Geometry: see drawing. Coordinates: mm, zero at the bounding-box minimum. Give positions to 0.01 mm unless a question says otherwise; leave off trailing zeros. Order: outer loops, then holes, each group sorted by start corner. A loop starts at its lowest first (then second) coordinate and runs counter-clockwise, first axis right, second up. Notation, with made-up numbers: M 2.5,74.25 L 12.5,74.25 A35 ccw 12.5,106.25 Z; hole C 39.25,12.25 d11. An arc over 180 degrees is marked long. Answer as a JSON object with one key per item and string values. Group by question number.
1. Section query C-C (x = 41.5). Output: boundary loops of the cut face in (y, z).
2. Material intervals for L1, parallel to X at y = 2.1, z = 21.5; L2, parallel to Z at x = 53.79, y = 0.9 (3 decimals); L3, parallel to Z at x = 26.5, y = 0.9, sorted ascending. Write a range as [from, to].
3. Section query A-A (x = 53.79). Output: boundary loops of the cut face in (y, z) (3 decimals).
4. Section query D-D (y = 1.7). Output: boundary loops of the cut face in (x, z) (3 decimals), plus the area to 3 significant figures.
5. Section query B-B (z = 6). Output: boundary loops of the cut face in (x, y).
6. Pin query (flat end, axial travel): P1, Ø1.6, axis at x = 22.5, y = 1, coming from the +Z side; P2, Ø1, axis at x = 32, y = 2, coming from the -Z side; P3, Ø1, axis at y = 1, z = 12, coming from the +X side. Return the tip coordinate at first contact, or that it passes through.
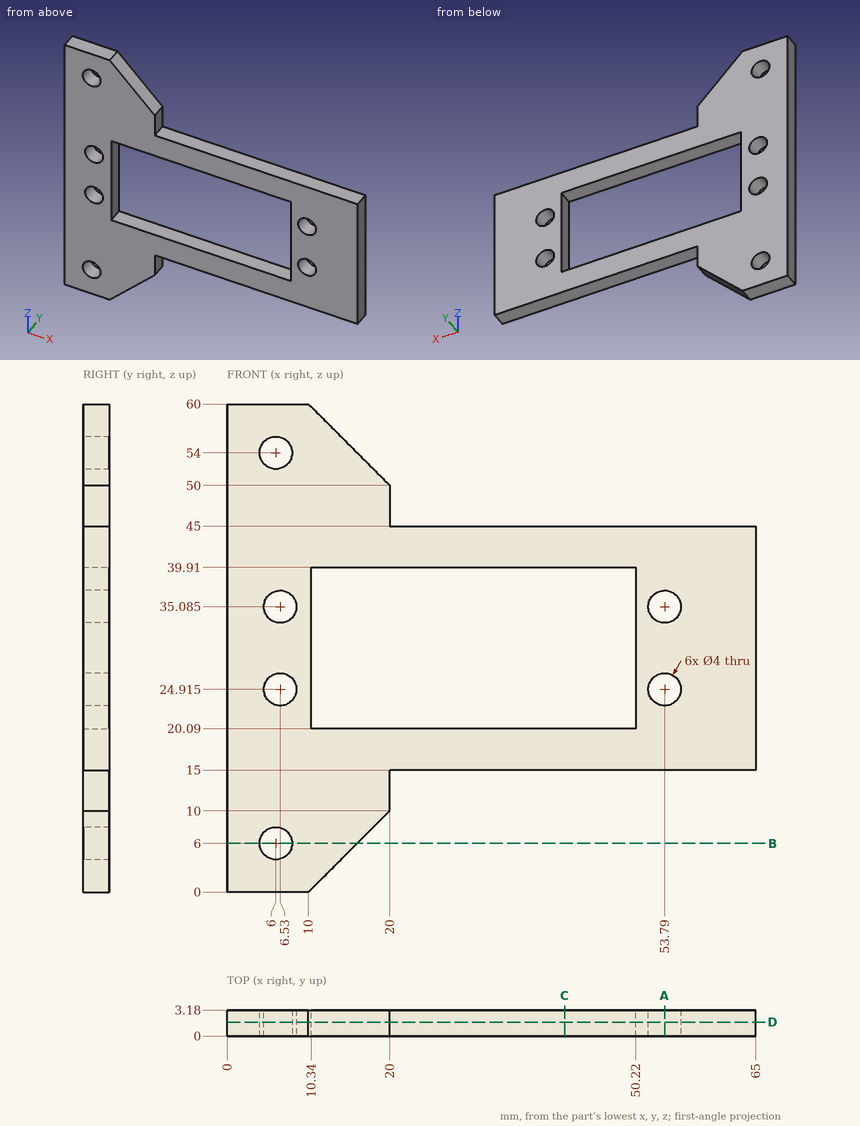
Answer sheet:
{
 "1": {"outline": "M 0,15 L 3.18,15 L 3.18,20.09 L 0,20.09 Z; M 0,39.91 L 3.18,39.91 L 3.18,45 L 0,45 Z"},
 "2": {"L1": "[0, 10.34], [50.22, 65]", "L2": "[15, 22.915], [26.915, 33.085], [37.085, 45]", "L3": "[15, 20.09], [39.91, 45]"},
 "3": {"outline": "M 0,15 L 3.18,15 L 3.18,22.915 L 0,22.915 Z; M 0,26.915 L 3.18,26.915 L 3.18,33.085 L 0,33.085 Z; M 0,37.085 L 3.18,37.085 L 3.18,45 L 0,45 Z"},
 "4": {"outline": "M 0,0 L 10,0 L 20,10 L 20,15 L 65,15 L 65,45 L 20,45 L 20,50 L 10,60 L 0,60 Z; hole C 6,6 d4; hole C 6,54 d4; hole C 6.53,24.915 d4; hole C 6.53,35.085 d4; hole M 10.34,20.09 L 50.22,20.09 L 50.22,39.91 L 10.34,39.91 Z; hole C 53.79,24.915 d4; hole C 53.79,35.085 d4", "area": "1,580 mm^2"},
 "5": {"outline": "M 0,0 L 4,0 L 4,3.18 L 0,3.18 Z; M 8,0 L 16,0 L 16,3.18 L 8,3.18 Z"},
 "6": {"P1": "z = 45", "P2": "z = 15", "P3": "x = 20"}
}
